```python
from build123d import *

# Parameters (mm, degrees)
BOSS_EXTRUDE1_DEPTH     = 27
SKETCH2_R               = 3.25
BOSS_EXTRUDE2_DEPTH     = 5
CUT_EXTRUDE1_DEPTH      = 92.228395409
CUT_EXTRUDE1_DEPTH_BACK = 92.228395409
SKETCH3_R               = 3.2
SKETCH4_W               = 10
SKETCH4_H               = 5
SKETCH4_H_2             = 3
CUT_EXTRUDE2_DEPTH      = 10.2
CUT_EXTRUDE3_DEPTH      = 90.058122159
CUT_EXTRUDE3_DEPTH_BACK = 90.058122159
SKETCH5_R               = 2.15
CUT_EXTRUDE4_DEPTH      = 92.183595829
CUT_EXTRUDE4_DEPTH_BACK = 92.183595829
SKETCH6_R               = 3.3
CUT_EXTRUDE5_START      = 9.55
SKETCH8_W               = 14
SKETCH8_H               = 14.4
CUT_EXTRUDE5_DEPTH      = 10
CUT_EXTRUDE6_START      = -7.45
SKETCH8_2_W             = 14
SKETCH8_2_H             = 14.4
CUT_EXTRUDE6_DEPTH      = 10
CUT_EXTRUDE7_DEPTH      = 87.332404543
CUT_EXTRUDE8_START      = -1
CUT_EXTRUDE8_DEPTH      = 86.163733723
FILLET3_R               = 5
FILLET4_R               = 2
FILLET5_R               = 0.3


with BuildPart() as part:
    # Sketch1 → Boss-Extrude1 (new body)
    with BuildSketch(Plane(origin=(0, 0, 0), x_dir=(1, 0, 0), z_dir=(0, 1, 0))):
        Polygon((0, 7.55), (-32.6, 7.55), (-49.874368671, 24.824368671), (-46.338834765, 28.359902577), (-30.428932188, 12.45), (75, 12.45), (75, -12.55), (-30.528932188, -12.55), (-46.338834765, -28.359902577), (-49.874368671, -24.824368671), (-32.6, -7.55), (0, -7.55), align=None)
    extrude(amount=BOSS_EXTRUDE1_DEPTH)

    # Sketch2 → Boss-Extrude2 (add)
    with BuildSketch(Plane(origin=(0, 27, 0), x_dir=(1, 0, 0), z_dir=(0, 1, 0))):
        Polygon((-49.874368671, 24.824368671), (-49.874368671, -24.824368671), (-46.338834765, -28.359902577), (-30.528932188, -12.55), (75, -12.55), (75, 12.45), (-30.428932188, 12.45), (-46.338834765, 28.359902577), align=None)
        with Locations(Location((-25, 0, 0), (0, 0, 270))):
            Circle(SKETCH2_R, mode=Mode.SUBTRACT)
    extrude(amount=BOSS_EXTRUDE2_DEPTH)

    # Sketch3 → Cut-Extrude1 (cut, two sides: drawn at the far end of the back side and taken through both)
    with BuildSketch(Plane.XY.offset(12.55).offset(-CUT_EXTRUDE1_DEPTH_BACK)):
        with Locations((-11, 17)):
            Circle(SKETCH3_R)
    extrude(amount=CUT_EXTRUDE1_DEPTH + CUT_EXTRUDE1_DEPTH_BACK, mode=Mode.SUBTRACT)

    # Sketch4 → Cut-Extrude2 (cut)
    with BuildSketch(Plane(origin=(0, 32, 0), x_dir=(1, 0, 0), z_dir=(0, 1, 0))):
        with Locations((23.58571545, 9.95)):
            Rectangle(SKETCH4_W, SKETCH4_H)
        with Locations((23.58571545, -11.05)):
            Rectangle(SKETCH4_W, SKETCH4_H_2)
    extrude(amount=-CUT_EXTRUDE2_DEPTH, mode=Mode.SUBTRACT)

    # Sketch5 → Cut-Extrude3 (cut, two sides: drawn at the far end of the back side and taken through both)
    with BuildSketch(Plane(origin=(0, 0, -7.45), x_dir=(-1, 0, 0), z_dir=(0, 0, -1)).offset(-CUT_EXTRUDE3_DEPTH_BACK)):
        with Locations((-23.58571545, 27)):
            Circle(SKETCH5_R)
    extrude(amount=CUT_EXTRUDE3_DEPTH + CUT_EXTRUDE3_DEPTH_BACK, mode=Mode.SUBTRACT)

    # Sketch6 → Cut-Extrude4 (cut, two sides: drawn at the far end of the back side and taken through both)
    with BuildSketch(Plane(origin=(0, 0, -12.45), x_dir=(-1, 0, 0), z_dir=(0, 0, -1)).offset(-CUT_EXTRUDE4_DEPTH_BACK)):
        with Locations((-60, 12.5)):
            Circle(SKETCH6_R)
    extrude(amount=CUT_EXTRUDE4_DEPTH + CUT_EXTRUDE4_DEPTH_BACK, mode=Mode.SUBTRACT)

    # Sketch8 → Cut-Extrude5 (cut)
    with BuildSketch(Plane.XY.offset(CUT_EXTRUDE5_START)):
        with Locations((23.58571545, 27)):
            Rectangle(SKETCH8_W, SKETCH8_H)
    extrude(amount=CUT_EXTRUDE5_DEPTH, mode=Mode.SUBTRACT)

    # Sketch8<2> → Cut-Extrude6 (cut)
    with BuildSketch(Plane.XY.offset(CUT_EXTRUDE6_START)):
        with Locations((23.58571545, 27)):
            Rectangle(SKETCH8_2_W, SKETCH8_2_H)
    extrude(amount=-CUT_EXTRUDE6_DEPTH, mode=Mode.SUBTRACT)

    # Sketch9 → Cut-Extrude7 (cut, through all)
    with BuildSketch(Plane.XZ):
        Polygon((75, 12.55), (47, 12.55), (47, 12.05), (74.5, 12.05), (74.5, -11.95), (47, -11.95), (47, -12.45), (75, -12.45), (75, -11.95), (75, 12.05), align=None)
    extrude(amount=-CUT_EXTRUDE7_DEPTH, mode=Mode.SUBTRACT)

    # Sketch10 → Cut-Extrude8 (cut, through all)
    with BuildSketch(Plane.XZ.offset(-27).offset(CUT_EXTRUDE8_START)):
        Polygon((-50.874368671, 27.238582233), (-50.874368671, -27.238582233), (-32.185786438, -8.55), (1, -8.55), (1, 8.55), (-32.185786438, 8.55), align=None)
    extrude(amount=CUT_EXTRUDE8_DEPTH, mode=Mode.SUBTRACT)

    # Fillet3
    fillet3_edges = [part.edges().sort_by_distance(p)[0] for p in [
        (-30.428932188, 16, -12.45),
        (-30.528932188, 16, 12.55),
    ]]
    fillet(fillet3_edges, radius=FILLET3_R)

    # Fillet4
    fillet4_edges = [part.edges().sort_by_distance(p)[0] for p in [
        (74.5, 16, 12.05),
        (74.5, 16, -11.95),
    ]]
    fillet(fillet4_edges, radius=FILLET4_R)

    # Fillet5
    fillet5_edges = [part.edges().sort_by_distance(p)[0] for p in [
        (47, 16, 12.55),
        (47, 16, -12.45),
    ]]
    fillet(fillet5_edges, radius=FILLET5_R)


solid = part.part
```
Input: part model. Units: mm. Frame: model coordinates. A direction names the side the tool comes from. Round coordinates to 2 decimals unless told otherwise and drop trailing zeros. Loops run counter-clockwise (first coordinate to the right, second up) from the corner with the lowest first, then second, coordinate; pieces in that order, holes last.
1) Material intervals for line 1 (Z direction, x = -7, y = 15); line 2 (X direction, y = 12.5, z = -1); line 3 (Y direction, x = -11, z = 9.9), sorted ascending.
Ans:
line 1: z = -12.45 to -8.55, 8.55 to 12.55
line 2: x = 1 to 56.7, 63.3 to 74.5
line 3: y = 0 to 13.8, 20.2 to 32
2) Pull-direction query (Y, two-part tool) for faces 5 (the flat face through (27, 0, -2)), 6 (the cylindrical face through (-11.694, 13.876, -10.527)), 7 (the cylindrical face through (62.619, 10.492, 0.218)), 8 (the flat face through (30.586, 26, 11)); classes: released by +Y, released by -Y, zero draft, split by the parting line, or undercut.
Ans:
face 5: released by -Y
face 6: undercut
face 7: undercut
face 8: zero draft
3) Set-up query: faces 1 (the flat face through (60, 16, 12.05)), 2 (the flat face through (-15, 14, 8.55)), 3 (the flat face through (16.586, 26, -10)), 4 (the flat face through (16.586, 26, 11)). Return all of +Z, -Z, +X, -X, +Y, -Y with unobstructed straight access to the full face (end or side cutting, diameter ignored); none if empty.
Ans:
face 1: +Z, +X, +Y, -Y
face 2: -X, -Y
face 3: -Z, +Y
face 4: +Z, +Y
4) Section query C-C on x = 60. Return the cut outline in (y, z), plus the area to 3 significant figures.
Ans:
outline: (0, -11.95) - (9.2, -11.95) - (9.2, 12.05) - (0, 12.05) - close; (15.8, -11.95) - (32, -11.95) - (32, 12.05) - (15.8, 12.05) - close
area: 610 mm2
5) Section query A-A on z = 0. Return the cut outline in (x, y), plus the area to 3 significant figures.
Ans:
outline: (-49.87, 28) - (-28.25, 28) - (-28.25, 32) - (-49.87, 32) - close; (-21.75, 28) - (1, 28) - (1, 0) - (74.5, 0) - (74.5, 32) - (-21.75, 32) - close; hole circle Ø4.3 at (23.59, 27); hole circle Ø6.6 at (60, 12.5)
area: 2,480 mm2
6) Pin query (flat end, axial travel): pin 1 (10 mm diameter, centred on x = 22, y = 23.5, fed in from -Z); pin 2 (10 mm diameter, centred on x = -18, z = 15.5, fed in from +Y); pin 3 (13 mm diameter, centred on x = 56, y = 8, fed in from -Z); pin 4 (4 mm diameter, centred on x = 3.5, y = 10.5, fed in from +Z). Return the tip coordinate at first contact, or that it passes through.
Ans:
pin 1: stops at z = -12.45
pin 2: stops at y = 32
pin 3: stops at z = -11.95
pin 4: stops at z = 12.55
7) Section query B-B on y = 17. Count the separate pieces of the cut face and the enclosed holes in it, plus the area to 3 significant figures.
Ans:
separate pieces: 3
enclosed holes: 0
area: 2,200 mm2
8) Section query D-D on z = 6.5. Return the cut outline in (x, y).
Ans:
outline: (-49.87, 28) - (1, 28) - (1, 0) - (74.5, 0) - (74.5, 32) - (-49.87, 32) - close; hole circle Ø4.3 at (23.59, 27); hole circle Ø6.6 at (60, 12.5)
